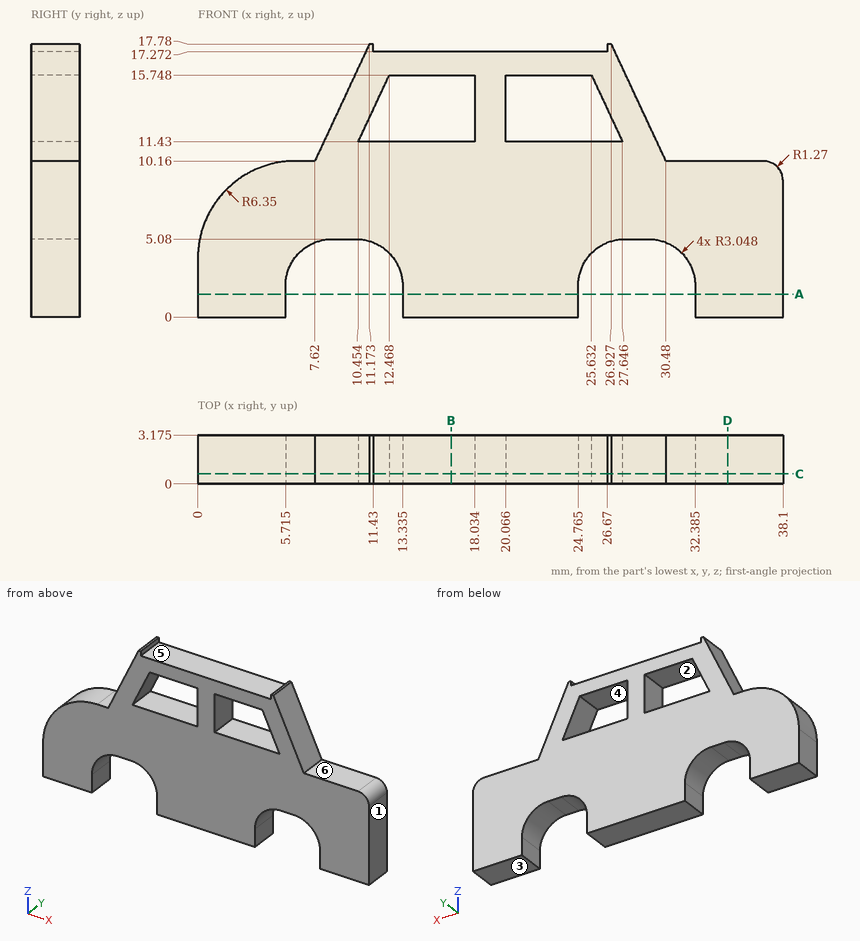
For this review, use the dimensioned drawing (mm, ordinates from the lowest corner) and the shaded views. A direction names the side the tool comes from. Give positions to 0.01 mm unless a question says otherwise; leave off trailing zeros. Order: outer loops, then holes, each group sorted by start corner. A loop starts at its lowest first (then second) coordinate and runs counter-clockwise, first axis right, second up.
1. Add section A-A, the plane z = 1.5. State the section outline as (x, y) points (1 decimal).
Solution:
outline: (0, 0) - (5.7, 0) - (5.7, 3.2) - (0, 3.2) - close; (13.3, 0) - (24.8, 0) - (24.8, 3.2) - (13.3, 3.2) - close; (32.4, 0) - (38.1, 0) - (38.1, 3.2) - (32.4, 3.2) - close
2. For pin 1 Ø1 at (y, z) = (2, 14.5) entering from -X; pin 2 Ø0.8 at (x, y) = (28.5, 1.5) entering from -Z; pin 3 Ø1 at (x, y) = (22.5, 1.5) entering from +Z, all flat-tipped, find the tip position at first contact; note any pin that passes through.
Solution:
pin 1: stops at x = 9.41
pin 2: stops at z = 5.08
pin 3: stops at z = 17.27
3. Add section D-D, the plane x = 34.5. State the section outline as (y, z) points (1 decimal).
Solution:
outline: (0, 0) - (3.2, 0) - (3.2, 10.2) - (0, 10.2) - close
4. Add section C-C, the plane y = 0.65. State how many separate pieces and enclosed holes the cut face has, then the cut area to 3 significant figures.
Solution:
separate pieces: 1
enclosed holes: 2
area: 391 mm2
5. To check wall thickness, follow L1, parallel to Z at x = 22, y = 1.85; L2, parallel to X at y = 1.55, z = 14 (1 decimal); L3, parallel to X at y = 1.6, z = 14.5 (1 decimal). State the ranges of each line that lie inside material, in increasing order.
Solution:
L1: z = 0 to 11.43, 15.75 to 17.27
L2: x = 9.4 to 11.7, 18 to 20.1, 26.4 to 28.7
L3: x = 9.6 to 11.9, 18 to 20.1, 26.2 to 28.5
6. Tool access review of the marked faces 4, 5 and 6: name each direction out of +Z, -Z, +X, -X, +Y, -Y from which nothing blocks a thin tool from reaching the whole face with its end or side.
Solution:
face 4: +Y, -Y
face 5: +Z, +Y, -Y
face 6: +Z, +X, +Y, -Y
7. Add section B-B, the plane x = 16.5. State the section outline as (y, z) points (1 decimal).
Solution:
outline: (0, 0) - (3.2, 0) - (3.2, 11.4) - (0, 11.4) - close; (0, 15.7) - (3.2, 15.7) - (3.2, 17.3) - (0, 17.3) - close
8. Mouldability with a two-part tool opening along X and no side actions: class the marked faces 1, 2 and 3 as +X half, -X half, draft (parallel to the pull), parting line (faces both ways), or undercut.
Solution:
face 1: +X half
face 2: undercut
face 3: draft
